Input: part model. Units: mm. Frame: model coordinates. Face numbers are marked on the shaded views. A direction names the side the tool comes from. Coordinates: 2 decimals unless noted, no trailing zeros. Write each loop counter-clockwise with the first axis right and the second up, starting at its lowest first coordinate (ties: lowest second). Pieces come first, ordered by that corner, then holes. Notation, with made-up numbers: M -2.5,-7 L 10.5,-7 A22 ccw 10.5,21 Z; hole C 54.5,-25.75 d3. An arc over 180 degrees is marked long. Use one line per item in the form item = value.
Solid Edge part; units mm, degrees
sketch "Sketch1" plane through (0, 0, 0) normal (0, 0, 1) x (1, 0, 0)
  line L0 (0, -4.0415) -> (3.5, -2.0207)
  line L1 (3.5, -2.0207) -> (3.5, 2.0207)
  line L2 (3.5, 2.0207) -> (0, 4.0415)
  line L3 (0, 4.0415) -> (-3.5, 2.0207)
  line L4 (-3.5, 2.0207) -> (-3.5, -2.0207)
  line L5 (-3.5, -2.0207) -> (0, -4.0415)
extrude "Protrusion1" add sketch "Sketch1" against normal blind 2.5
sketch "Sketch2" plane through (0, 0, -2.5) normal (0, 0, -1) x (0.866, 0.5, 0)
  circle A0 centre (0, 0) radius 5
extrude "ExtrudedProtrusion_2" add sketch "Sketch2" along normal blind 0.5
sketch "Sketch3" plane through (0, 0, -2.5) normal (0, 0, -1) x (0.866, 0.5, 0)
  circle A0 centre (0, 0) radius 2.5
extrude "ExtrudedProtrusion_3" add sketch "Sketch3" along normal blind 10
sketch "Sketch4" plane through (0, 0, 0) normal (0, -1, 0) x (1, 0, 0)
  line L0 (6.9641, 0) -> (3.5, 0)
  line L1 (3.5, 0) -> (6.9641, -2)
  line L2 (6.9641, -2) -> (6.9641, 0)
revolve "RevolvedCutout1" cut sketch "Sketch4" angle 90 about axis through (0, 0, 0) along (0, 0, -1)
sketch "Sketch5" plane through (0, 0, 0) normal (0, -1, 0) x (1, 0, 0)
  line L0 (3.1642, 0.1939) -> (4.2543, 0.1939)
  line L1 (4.2543, 0.1939) -> (4.2543, -0.4355)
  line L2 (4.2543, -0.4355) -> (3.5, 0)
  line L3 (3.5, 0) -> (3.1642, 0.1939)
revolve "RevolvedCutout_6" cut sketch "Sketch5" angle 90 about axis through (0, 0, 0) along (0, 0, 1)
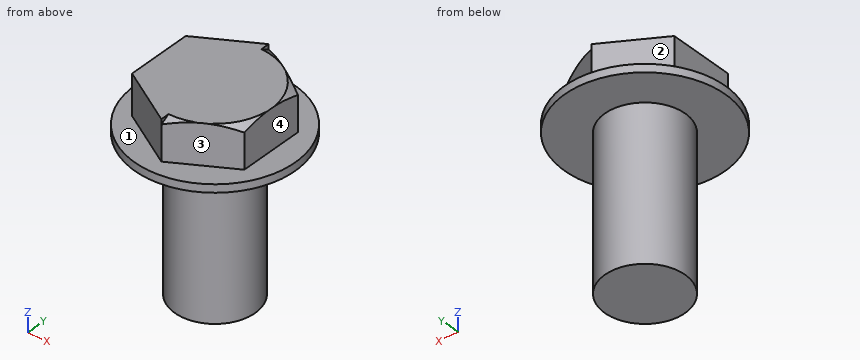
(1) Line query: probe 1 along Z at (x, y) = (-2.5, 2.25); probe 2 along Z at (x, y) = (3, 3); probe 3 along X at (y, z) = (-2.25, -1.75). Output: solid intervals per line, ascending.
Computed:
probe_1 = -3 to 0
probe_2 = -3 to -2.5
probe_3 = -3.1 to 3.1
(2) Section query B-B on z = -9.5. Return the cut outline in (x, y), plus the area to 3 significant figures.
Computed:
outline = C 0,0 d5
area = 19.6 mm^2
(3) Set-up query: the marked faces 1, 2, 3 and 4. Return all of +Z, -Z, +X, -X, +Y, -Y with unobstructed straight access to the full face (end or side cutting, diameter ignored); none if empty.
Computed:
face_1 = +Z
face_2 = +Z, -X, +Y
face_3 = +Z, +X, -Y
face_4 = +Z, +X, +Y, -Y
(4) First-contact query: pin 1 Ø6 at (x, z) = (3, -1.5) entering from +Y; pin 2 Ø3 at (y, z) = (0.5, -1.5) entering from +X; pin 3 Ø1 at (y, z) = (-2.5, -11) entering from +X; pin 4 Ø3 at (y, z) = (-0.5, -0.5) entering from -X. Flat tips, straight axial feed; report the tip coordinate or a pass-through.
Computed:
pin_1 = 5
pin_2 = 5
pin_3 = 1.5
pin_4 = -3.5
(5) Section query A-A on x = -1. Return the cut outline in (y, z), plus the area to 3 significant figures.
Computed:
outline = M -4.9,-3 L -2.29,-3 L -2.29,-12.5 L 2.29,-12.5 L 2.29,-3 L 4.9,-3 L 4.9,-2.5 L 3.46,-2.5 L 3.46,0 L -3.46,0 L -3.46,-2.5 L -4.9,-2.5 Z
area = 65.8 mm^2
